from build123d import *

# Parameters (mm, degrees)
F0_W     = 60
F0_H     = 15
F1_DEPTH = 5
F2_W     = 60
F2_H     = 13
F3_DEPTH = 15
F5_D     = 4.2
F5_DEPTH = 10.4
F5_TIP   = 1.2618073
F7_D     = 4.2
F7_DEPTH = 8
F7_TIP   = 1.2618073
F8_SIZE  = 1


with BuildPart() as f1:
    # F0 (on Top) → F1 (new body)
    with BuildSketch(Plane.XY):
        with Locations((30, 7.5)):
            Rectangle(F0_W, F0_H)
    extrude(amount=F1_DEPTH)

    # F2 (on face) → F3 (join)
    with BuildSketch(Plane.XY.offset(5)):
        with Locations((30, 6.5)):
            Rectangle(F2_W, F2_H)
    extrude(amount=F3_DEPTH)

    # F5
    with Locations(Plane.YZ.offset(60)):
        with Locations((7.5, 10)):
            Hole(F5_D / 2, depth=F5_DEPTH)
            with Locations((0, 0, -(F5_DEPTH + F5_TIP / 2))):  # 118° drill point
                Cone(0, F5_D / 2, F5_TIP, mode=Mode.SUBTRACT)

    # F7
    with Locations(Plane(origin=(0, 0, 0), x_dir=(0, -1, 0), z_dir=(-1, 0, 0))):
        with Locations((-7.5, 10)):
            Hole(F7_D / 2, depth=F7_DEPTH)
            with Locations((0, 0, -(F7_DEPTH + F7_TIP / 2))):  # 118° drill point
                Cone(0, F7_D / 2, F7_TIP, mode=Mode.SUBTRACT)

    # F8
    f8_edges = [f1.edges().sort_by_distance(p)[0] for p in [
        (30, 13, 20),
        (30, 0, 20),
        (0, 6.5, 20),
        (60, 6.5, 20),
    ]]
    chamfer(f8_edges, length=F8_SIZE)


solid = f1.part
CAD build for the part. Positions are in the model's coordinates, mm. A direction names the side the tool comes from. Round coordinates to 2 decimals unless told otherwise and drop trailing zeros. Order: outer loops, then holes, each group sorted by start corner. A loop starts at its lowest first (then second) coordinate and runs counter-clockwise, first axis right, second up. Notation, with made-up numbers: (84, -26) - (96, -26) arc R27 ccw to (96, -4) - close; hole circle Ø11 at (44.25, 45). An arc over 180 degrees is marked (long way). Return JSON: item names as keys, results as strings.
(1) Cut at A-A (x = 21.5). Give the cut face in (y, z).
Answer key:
{"outline": "(0, 0) - (15, 0) - (15, 5) - (13, 5) - (13, 19) - (12, 20) - (1, 20) - (0, 19) - close"}
(2) Pin check, flat tips, straight feed: pin 1 Ø2.5 at (y, z) = (7.5, 10) entering from -X; pin 2 Ø1 at (x, y) = (40, 14) entering from +Z. Stop position of each tip, or through.
Answer key:
{"pin 1": "stops at x = 8.51", "pin 2": "stops at z = 5"}
(3) Wall check: probe 1 along Z at (x, y) = (56.25, 7.5); probe 2 along Y at (x, z) = (52.25, 10); probe 3 along Z at (x, y) = (57.5, 13.25). Give the ranges that are in metal, low to high. Write a range as from..to.
Answer key:
{"probe 1": "z = 0..7.9, 12.1..20", "probe 2": "y = 0..5.4, 9.6..13", "probe 3": "z = 0..5"}
(4) Pull direction Y, two halves, no side cores. Call faces 6 (the face through (30, 7, 20)), 7 (the face through (30, 0, 9)), 8 (the face through (48.557, 7.453, 10.362)): +Y half, -Y half, draft (parallel to the pull), parting line (faces both ways), or undercut.
Answer key:
{"face 6": "draft", "face 7": "-Y half", "face 8": "undercut"}
(5) Cut at C-C (y = 14.25). Give the cut face in (x, z).
Answer key:
{"outline": "(0, 0) - (60, 0) - (60, 5) - (0, 5) - close"}
(6) Cut at B-B (z = 6.5). Give the cut face in (x, y).
Answer key:
{"outline": "(0, 0) - (60, 0) - (60, 13) - (0, 13) - close"}
(7) Tool access for faces 1 (the face through (54.727, 7.773, 12.082)), 2 (the face through (30, 14, 5)), 3 (the face through (4.056, 7.227, 12.082)), 4 (the face through (60, 7, 7)), 5 (the face through (0, 7, 7)): list every direction of +Z, -Z, +X, -X, +Y, -Y with a clear straight run to the whole face (end or side of a thin tool).
Answer key:
{"face 1": "+X", "face 2": "+Z, +X, -X, +Y", "face 3": "-X", "face 4": "+Z, -Z, +X, +Y, -Y", "face 5": "+Z, -Z, -X, +Y, -Y"}
